Build history of the part. All positions in model axes, mm. A direction names the side the tool comes from. Round coordinates to 2 decimals unless told otherwise and drop trailing zeros. Write each loop counter-clockwise with the first axis right and the second up, starting at its lowest first coordinate (ties: lowest second). Pieces come first, ordered by that corner, then holes. Notation, with made-up numbers: (77.5, 4) - (133.5, 4) arc R11 ccw to (133.5, 12) - close; hole circle Ø2 at (-10, 74). An arc over 180 degrees is marked (long way). One line per question, with ' | ' between items.
from build123d import *

# Parameters (mm, degrees)
F0_W   = 16.2657573819
F0_H   = 3.7642940879
F0_W_2 = 15.1902455837
F0_H_2 = 9.9756410345


with BuildPart() as f1:
    # F0 (on Front) → F1 (revolve)
    with BuildSketch(Plane.XZ):
        Polygon((0, 38.4767018259), (0, 55.9537671506), (-34.8183326423, 55.9537671506), (-34.8183326423, 38.4767018259), (-28.9030186832, 38.4767018259), align=None)
        Polygon((0, 20.7307580858), (0, 38.4767018259), (-28.9030186832, 38.4767018259), (-28.9030186832, 20.7307580858), (-21.1055595428, 20.7307580858), align=None)
        with Locations((-8.132878691, -68.5367174447)):
            Rectangle(F0_W, F0_H)
        Polygon((0, -66.6545704007), (0, 0), (-15.1902455837, 0), (-22.4499497563, 0), (-22.4499497563, -66.6545704007), (-16.2657573819, -66.6545704007), align=None)
        with Locations((-7.5951227918, 4.9878205173)):
            Rectangle(F0_W_2, F0_H_2)
        Polygon((0, 9.9756410345), (0, 20.7307580858), (-21.1055595428, 20.7307580858), (-21.1055595428, 9.9756410345), (-15.1902455837, 9.9756410345), align=None)
    revolve(axis=Axis((0, 0, -74.1831511259), (0, 0, -1)))


solid = f1.part
Q1. Saw through at B-B, the plane y = 0. List the corners of the cut face in (x, z).
Found:
outline: (-34.82, 38.48) - (-28.9, 38.48) - (-28.9, 20.73) - (-21.11, 20.73) - (-21.11, 9.98) - (-15.19, 9.98) - (-15.19, 0) - (-22.45, 0) - (-22.45, -66.65) - (-16.27, -66.65) - (-16.27, -70.42) - (16.27, -70.42) - (16.27, -66.65) - (22.45, -66.65) - (22.45, 0) - (15.19, 0) - (15.19, 9.98) - (21.11, 9.98) - (21.11, 20.73) - (28.9, 20.73) - (28.9, 38.48) - (34.82, 38.48) - (34.82, 55.95) - (-34.82, 55.95) - close
Q2. Drop flat-ended pins along their axis: pin 1 (2 mm diameter, centred on x = -11.5, y = -24.5, fed in from -Z); pin 2 (1.5 mm diameter, centred on y = -13, z = -42, fed in from -X); pin 3 (8 mm diameter, centred on x = -19.5, z = 41, fed in from -Y). Give the stop position or say it passes through.
Found:
pin 1: z = 20.73 | pin 2: x = -18.81 | pin 3: y = -31.18
Q3. Saw through at A-A, the plane y = -19.5. List the corners of the cut face in (x, z), then the cut area to 3 significant figures.
Found:
outline: (-28.85, 38.48) - (-21.33, 38.48) - (-21.33, 20.73) - (-8.07, 20.73) - (-8.07, 9.98) - (8.07, 9.98) - (8.07, 20.73) - (21.33, 20.73) - (21.33, 38.48) - (28.85, 38.48) - (28.85, 55.95) - (-28.85, 55.95) - close; (-11.12, -66.65) - (11.12, -66.65) - (11.12, 0) - (-11.12, 0) - close | area: 3,420 mm^2
Q4. Saw through at D-D, the plane z = -53.5. List the corners of the cut face in (x, y).
Found:
outline: circle Ø44.9 at (0, 0)
Q5. Drill centre lines: L1, parallel to Z at x = 15.5, y = -13; L2, parallel to Z at x = 26.5, y = 20; L3, parallel to Z at x = -26, y = 4. Where is each one in solid material? Low to high. Write a range as from..to.
Found:
L1: -66.65..0, 9.98..55.95 | L2: 38.48..55.95 | L3: 20.73..55.95
Q6. Which spindle directions (+Z, -Z, +X, -X, +Y, -Y) get a long thin tool onto all of the face, cutting with end or side? Do faces 1 (the flat face through (0, 0, -70.419)), 2 (the cylindrical face through (12.054, -9.243, 5.058)), 3 (the flat face through (-15, 7, -66.655)). Say none if no direction does.
Found:
face 1: -Z, +X, -X, +Y, -Y | face 2: none | face 3: -Z
